from build123d import *

# Parameters (mm, degrees)
CROQUIS1_W                = 5.9
CROQUIS1_H                = 10
CROQUIS1_R                = 1.75
SALIENTE_EXTRUIR1_DEPTH   = 10
SALIENTE_EXTRUIR1_2_DEPTH = 10
SALIENTE_EXTRUIR2_DEPTH   = 10


with BuildPart() as part:
    # Croquis1 → Saliente-Extruir1 (new body)
    with BuildSketch(Plane.XY):
        with Locations((-9.508333333, 2.425)):
            Rectangle(CROQUIS1_W, CROQUIS1_H)
        with Locations((-9.483333333, 2.425)):
            Circle(CROQUIS1_R, mode=Mode.SUBTRACT)
    extrude(amount=SALIENTE_EXTRUIR1_DEPTH)



with BuildPart() as body_2:
    # Croquis1 → Saliente-Extruir1 2 (new body)
    with BuildSketch(Plane.XY):
        with Locations((4.591666667, 2.425)):
            Rectangle(CROQUIS1_W, CROQUIS1_H)
        with Locations(Location((4.566666667, 2.425, 0), (0, 0, 180))):
            Circle(CROQUIS1_R, mode=Mode.SUBTRACT)
    extrude(amount=SALIENTE_EXTRUIR1_2_DEPTH)


with BuildPart() as part_1:
    add(part.part)

    add(body_2.part)  # Saliente-Extruir2 merges body 2
    # Croquis3 → Saliente-Extruir2 (add)
    with BuildSketch(Plane.XZ.offset(2.575)):
        with BuildLine():
            Line((-6.558333333, 10), (-6.558333333, 0))
            Line((-6.558333333, 0), (1.641666667, 0))
            Line((1.641666667, 0), (1.641666667, 10))
            ThreePointArc((1.641666667, 10), (-2.458333333, 5.9), (-6.558333333, 10))
        make_face()
    extrude(amount=-SALIENTE_EXTRUIR2_DEPTH)


solid = part_1.part
Source: CAD feature listing. Evaluate the final solid. Frame: model axes, mm. Coordinates: 2 decimals unless noted, no trailing zeros. Order: outer loops, then holes, each group sorted by start corner. A loop starts at its lowest first (then second) coordinate and runs counter-clockwise, first axis right, second up. Notation, with made-up numbers: M 79.25,70.5 L 121.25,70.5 A26 cw 121.25,107.5 Z; hole C 79.5,76.5 d5. An arc over 180 degrees is marked long. Write each question's results on one line, items separated by ' | '. Start each with the question number.
Item 1: Line query: probe 1 along X at (y, z) = (1.75, 5); probe 2 along X at (y, z) = (2, 9.25); probe 3 along X at (y, z) = (5.5, 8.75). Output: solid intervals per line, ascending.
Item 2: First-contact query: pin 1 Ø1.5 at (x, y) = (-7, 3.5) entering from -Z; pin 2 Ø1 at (x, y) = (-2.5, 2.5) entering from +Z. Flat tips, straight axial feed; report the tip coordinate or a pass-through.
Item 3: Cut plane D-D (y = 3.75). Return loops of the section in (x, z), and give its area (3 significant figures).
Item 4: Draft query along Y for faces 1 (the face through (3, 4, 10)), 2 (the face through (-8.68, 0.87, 4.93)), 3 (the face through (-3, 7.425, 5)). Return one class per face: pulls with the +Y half, pulls with the -Y half, needs draft (parallel to the pull), parting line crosses it, or undercut.
Item 5: Cut plane B-B (x = -9.25). Return loops of the section in (y, z) (3 decimals), and give its area (3 significant figures).
Item 6: Cut plane C-C (y = -1.5). Return loops of the section in (x, z), and give its area (3 significant figures).
Item 7: Cut plane A-A (z = 8). Return loops of the section in (x, y) (3 decimals).
Checked values:
1) probe 1: x = -12.46 to -11.1, -7.87 to 2.95, 6.18 to 7.54 | probe 2: x = -12.46 to -11.18, -7.79 to -6.49, 1.57 to 2.87, 6.26 to 7.54 | probe 3: x = -12.46 to -6.36, 1.45 to 7.54
2) pin 1: stops at z = 0 | pin 2: stops at z = 5.94
3) outline: M -12.46,0 L -10.63,0 L -10.63,10 L -12.46,10 Z; M -8.34,0 L 3.42,0 L 3.42,10 L 1.64,10 A4.1 cw -6.56,10 L -8.34,10 Z; M 5.71,0 L 7.54,0 L 7.54,10 L 5.71,10 Z | area: 128 mm2
4) face 1: needs draft | face 2: undercut | face 3: pulls with the +Y half
5) outline: M -2.575,0 L 0.691,0 L 0.691,10 L -2.575,10 Z; M 4.159,0 L 7.425,0 L 7.425,10 L 4.159,10 Z | area: 65.3 mm2
6) outline: M -12.46,0 L 7.54,0 L 7.54,10 L 1.64,10 A4.1 cw -6.56,10 L -12.46,10 Z | area: 174 mm2
7) outline: M -12.458,-2.575 L -6.037,-2.575 L -6.037,7.425 L -12.458,7.425 Z; M 1.121,-2.575 L 7.542,-2.575 L 7.542,7.425 L 1.121,7.425 Z; hole C -9.483,2.425 d3.5; hole C 4.567,2.425 d3.5
